Input: dimensioned drawing with shaded views. Units: mm. Origin: part minimum x, y, z. Give positions to 0.01 mm unless a question says otherwise; leave off trailing zeros. Write each loop counter-clockwise with the first axis right and the second up, starting at its lowest first coordinate (ties: lowest second). Pieces come first, ordered by that corner, then holes.
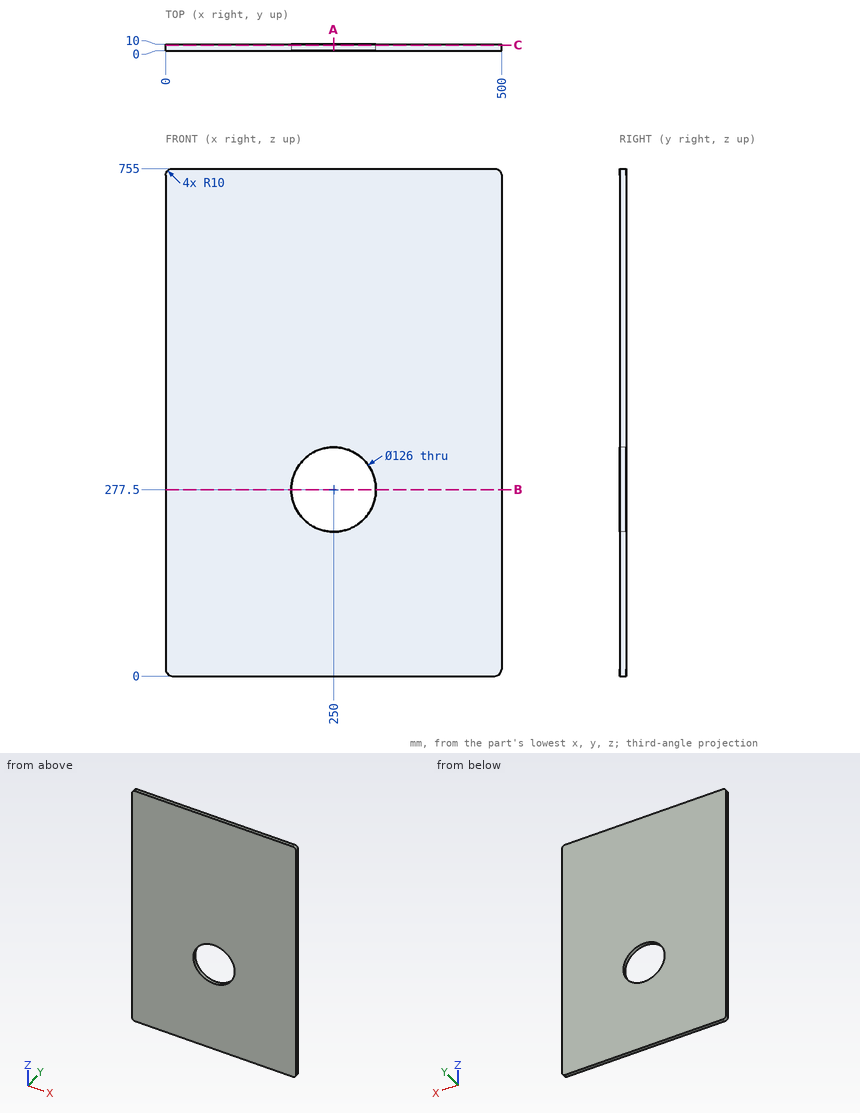
Item 1: Section C-C, the plane y = 8.5. Return the cut outline in (x, z).
Found:
outline: (0, 10) arc R10 ccw to (10, 0) - (490, 0) arc R10 ccw to (500, 10) - (500, 745) arc R10 ccw to (490, 755) - (10, 755) arc R10 ccw to (0, 745) - close; hole circle Ø126 at (250, 277.5)
Item 2: Line query: L1, parallel to Z at x = 250, y = 7.75; L2, parallel to X at y = 2.75, z = 277.5; L3, parallel to X at y = 3.5, z = 266. Output: solid intervals per line, ascending.
Found:
L1: z = 0 to 214.5, 340.5 to 755
L2: x = 0 to 187, 313 to 500
L3: x = 0 to 188.06, 311.94 to 500
Item 3: Section A-A, the plane x = 250. Return the cut outline in (y, z), plus the area to 3 significant figures.
Found:
outline: (0, 0) - (10, 0) - (10, 214.5) - (0, 214.5) - close; (0, 340.5) - (10, 340.5) - (10, 755) - (0, 755) - close
area: 6,290 mm2
Item 4: Section B-B, the plane z = 277.5. Return the cut outline in (x, y), plus the area to 3 significant figures.
Found:
outline: (0, 0) - (187, 0) - (187, 10) - (0, 10) - close; (313, 0) - (500, 0) - (500, 10) - (313, 10) - close
area: 3,740 mm2
